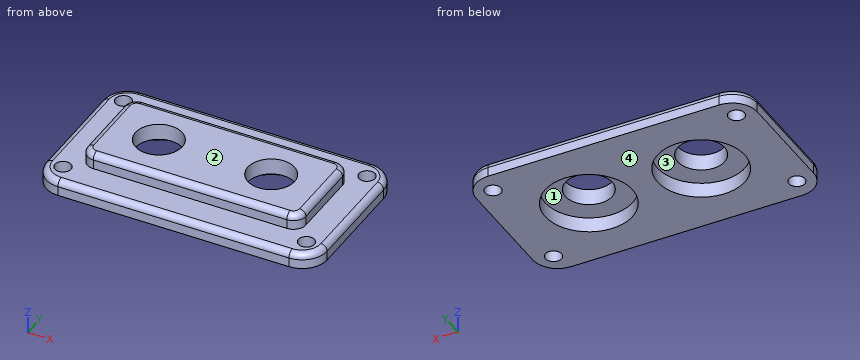
from build123d import *

# Parameters (mm, degrees)
F0_R     = 1.651
F0_R_2   = 4.7625
F1_DEPTH = 3.175
F2_DEPTH = 3.175
F3_R     = 1.27
F4_R     = 8.89
F5_DEPTH = 3.048


with BuildPart() as f1:
    # F0 (on Top) → F1 (new body)
    with BuildSketch(Plane.XY):
        with BuildLine():
            Line((-23.495, -15.875), (23.495, -15.875))
            ThreePointArc((23.495, -15.875), (27.087102, -14.387102), (28.575, -10.795))
            Line((28.575, -10.795), (28.575, 10.795))
            ThreePointArc((28.575, 10.795), (27.087102, 14.387102), (23.495, 15.875))
            Line((23.495, 15.875), (-23.495, 15.875))
            ThreePointArc((-23.495, 15.875), (-27.087102, 14.387102), (-28.575, 10.795))
            Line((-28.575, 10.795), (-28.575, -10.795))
            ThreePointArc((-28.575, -10.795), (-27.087102, -14.387102), (-23.495, -15.875))
        make_face()
        with Locations((-24.765, -11.557)):
            Circle(F0_R, mode=Mode.SUBTRACT)
        with Locations((24.765, -11.557)):
            Circle(F0_R, mode=Mode.SUBTRACT)
        with Locations((-24.765, 11.557)):
            Circle(F0_R, mode=Mode.SUBTRACT)
        with BuildLine():
            Line((-19.685, 9.525), (19.685, 9.525))
            ThreePointArc((19.685, 9.525), (21.481051, 8.781051), (22.225, 6.985))
            Line((22.225, 6.985), (22.225, -6.985))
            ThreePointArc((22.225, -6.985), (21.481051, -8.781051), (19.685, -9.525))
            Line((19.685, -9.525), (-19.685, -9.525))
            ThreePointArc((-19.685, -9.525), (-21.481051, -8.781051), (-22.225, -6.985))
            Line((-22.225, -6.985), (-22.225, 6.985))
            ThreePointArc((-22.225, 6.985), (-21.481051, 8.781051), (-19.685, 9.525))
        make_face(mode=Mode.SUBTRACT)
        with Locations((24.765, 11.557)):
            Circle(F0_R, mode=Mode.SUBTRACT)
        with BuildLine():
            ThreePointArc((22.225, 6.985), (21.481051, 8.781051), (19.685, 9.525))
            Line((19.685, 9.525), (-19.685, 9.525))
            ThreePointArc((-19.685, 9.525), (-21.481051, 8.781051), (-22.225, 6.985))
            Line((-22.225, 6.985), (-22.225, -6.985))
            ThreePointArc((-22.225, -6.985), (-21.481051, -8.781051), (-19.685, -9.525))
            Line((-19.685, -9.525), (19.685, -9.525))
            ThreePointArc((19.685, -9.525), (21.481051, -8.781051), (22.225, -6.985))
            Line((22.225, -6.985), (22.225, 6.985))
        make_face()
        with Locations((-11.43, 0)):
            Circle(F0_R_2, mode=Mode.SUBTRACT)
        with Locations((11.43, 0)):
            Circle(F0_R_2, mode=Mode.SUBTRACT)
    extrude(amount=-F1_DEPTH)

    # F0 (on Top) → F2 (join)
    with BuildSketch(Plane.XY):
        with BuildLine():
            ThreePointArc((22.225, 6.985), (21.481051, 8.781051), (19.685, 9.525))
            Line((19.685, 9.525), (-19.685, 9.525))
            ThreePointArc((-19.685, 9.525), (-21.481051, 8.781051), (-22.225, 6.985))
            Line((-22.225, 6.985), (-22.225, -6.985))
            ThreePointArc((-22.225, -6.985), (-21.481051, -8.781051), (-19.685, -9.525))
            Line((-19.685, -9.525), (19.685, -9.525))
            ThreePointArc((19.685, -9.525), (21.481051, -8.781051), (22.225, -6.985))
            Line((22.225, -6.985), (22.225, 6.985))
        make_face()
        with Locations((-11.43, 0)):
            Circle(F0_R_2, mode=Mode.SUBTRACT)
        with Locations((11.43, 0)):
            Circle(F0_R_2, mode=Mode.SUBTRACT)
    extrude(amount=F2_DEPTH)

    # F3
    f3_edges = [f1.edges().sort_by_distance(p)[0] for p in [
        (0, 9.525, 3.175),
        (0, 15.875, 0),
    ]]
    fillet(f3_edges, radius=F3_R)

    # F4 (on face) → F5 (cut)
    with BuildSketch(Plane(origin=(0, 0, -3.175), x_dir=(1, 0, 0), z_dir=(0, 0, -1))):
        with Locations((-11.43, 0)):
            Circle(F4_R)
        with Locations((11.43, 0)):
            Circle(F4_R)
    extrude(amount=-F5_DEPTH, mode=Mode.SUBTRACT)


solid = f1.part
Can you work these out from the model? Positions are in its coordinate system, mm. Face numbers are marked on the shaded views. A direction names the side the tool comes from. Round coordinates to 2 decimals unless told otherwise and drop trailing zeros. Write each loop counter-clockwise with the first axis right and the second up, starting at its lowest first coordinate (ties: lowest second). Pieces come first, ordered by that corner, then holes. Notation, with made-up numbers: M 34.5,79.5 L 61.5,79.5 A26 ccw 61.5,118.5 Z; hole C -34,-34 d3. An arc over 180 degrees is marked long. Use a Markdown table: item, result.
Item 1: I want a section at B-B (x = -11.43). List the corners of the cut face in (y, z) for me (1 decimal).
Found:
| item | result |
|---|---|
| outline | M -15.9,-3.2 L -8.9,-3.2 L -8.9,-0.1 L -4.8,-0.1 L -4.8,3.2 L -8.3,3.2 A1.3 ccw -9.5,1.9 L -9.5,0 L -14.6,0 A1.3 ccw -15.9,-1.3 Z; M 4.8,-0.1 L 8.9,-0.1 L 8.9,-3.2 L 15.9,-3.2 L 15.9,-1.3 A1.3 ccw 14.6,0 L 9.5,0 L 9.5,1.9 A1.3 ccw 8.3,3.2 L 4.8,3.2 Z |
Item 2: If I drill on line 1 along X through (y, z) = (0, -2.25) (3 decimals); line 2 along X through (y, z) = (0, 1.75) (1 decimal); line 3 along Y through (x, z) = (11.43, -2.05) (3 decimals), over which ranges is the centre line in solid material (lowest first)? Write a range as [from, to].
Found:
| item | result |
|---|---|
| line 1 | x = [-28.575, -20.32], [-2.54, 2.54], [20.32, 28.575] |
| line 2 | x = [-22.2, -16.2], [-6.7, 6.7], [16.2, 22.2] |
| line 3 | y = [-15.875, -8.89], [8.89, 15.875] |
Item 3: I want a section at D-D (z = -2.25). List the corners of the cut face in (x, y) for me (3 decimals).
Found:
| item | result |
|---|---|
| outline | M -28.575,-10.795 A5.08 ccw -23.495,-15.875 L 23.495,-15.875 A5.08 ccw 28.575,-10.795 L 28.575,10.795 A5.08 ccw 23.495,15.875 L -23.495,15.875 A5.08 ccw -28.575,10.795 Z; hole C -24.765,-11.557 d3.302; hole C -24.765,11.557 d3.302; hole C -11.43,0 d17.78; hole C 11.43,0 d17.78; hole C 24.765,-11.557 d3.302; hole C 24.765,11.557 d3.302 |
Item 4: Which directions (+Z, -Z, +X, -X, +Y, -Y) give clear straight access to the entire face, cutting with the end or side of a thin tool? Please do the marked faces 3 and 4.
Found:
| item | result |
|---|---|
| face 3 | -Z |
| face 4 | -Z, +X, -X, +Y, -Y |
Item 5: I want a section at C-C (z = 0.75). List the corners of the cut face in (x, y) for me (1 decimal), and give its area (3 significant figures).
Found:
| item | result |
|---|---|
| outline | M -22.2,-7 A2.5 ccw -19.7,-9.5 L 19.7,-9.5 A2.5 ccw 22.2,-7 L 22.2,7 A2.5 ccw 19.7,9.5 L -19.7,9.5 A2.5 ccw -22.2,7 Z; hole C -11.4,0 d9.5; hole C 11.4,0 d9.5 |
| area | 699 mm2 |
Item 6: I want a section at A-A (y = 0). List the corners of the cut face in (x, z) for me (1 decimal).
Found:
| item | result |
|---|---|
| outline | M -28.6,-3.2 L -20.3,-3.2 L -20.3,-0.1 L -16.2,-0.1 L -16.2,3.2 L -21,3.2 A1.3 ccw -22.2,1.9 L -22.2,0 L -27.3,0 A1.3 ccw -28.6,-1.3 Z; M -6.7,-0.1 L -2.5,-0.1 L -2.5,-3.2 L 2.5,-3.2 L 2.5,-0.1 L 6.7,-0.1 L 6.7,3.2 L -6.7,3.2 Z; M 16.2,-0.1 L 20.3,-0.1 L 20.3,-3.2 L 28.6,-3.2 L 28.6,-1.3 A1.3 ccw 27.3,0 L 22.2,0 L 22.2,1.9 A1.3 ccw 21,3.2 L 16.2,3.2 Z |
Item 7: We'd pull the mould along X, two halves only. Please class the marked faces 1 and 2: released by +X, released by -X, zero draft, split by the parting line, or undercut.
Found:
| item | result |
|---|---|
| face 1 | undercut |
| face 2 | zero draft |
Item 8: For pin 1 Ø0.6 at (x, z) = (1.5, 1) entering from -Y (3 decimals); pin 2 Ø12.5 at (x, y) = (11.43, 0) entering from -Z; pin 3 Ø0.6 at (y, z) = (-1.5, 0.5) entering from +X (3 decimals), each with a flat end and sliding along its axis, tell me the tip position at first contact or that it passes through.
Found:
| item | result |
|---|---|
| pin 1 | stops at y = -9.525 |
| pin 2 | stops at z = -0.13 |
| pin 3 | stops at x = 22.225 |
